Part model, mm, in its own coordinate system. A direction names the side the tool comes from. Give positions to 0.01 mm unless a question says otherwise; leave off trailing zeros. Loops run counter-clockwise (first coordinate to the right, second up) from the corner with the lowest first, then second, coordinate; pieces in that order, holes last. Notation, with made-up numbers: M 68,89.5 L 75,89.5 A22 ccw 75,125.5 Z; hole C 77.25,24 d7. An arc over 180 degrees is marked long. Put each result on its own line as item: value. Start each with the question number.
```python
from build123d import *

# Parameters (mm, degrees)
F1_DEPTH = 4


with BuildPart() as f1:
    # F0 (on Top) → F1 (new body)
    with BuildSketch(Plane.XY):
        with BuildLine():
            ThreePointArc((-21.3281772584, 26.4835794998), (-23.5728167331, 28.3513270209), (-20.7305210084, 27.6818181058))
            ThreePointArc((-20.7305210084, 27.6818181058), (-20.7359422147, 27.5544044904), (-20.7521666475, 27.4279118558))
            Line((-20.7521666475, 27.4279118558), (-19.7434481071, 27.4279118558))
            ThreePointArc((-19.7434481071, 27.4279118558), (-19.7337548746, 27.5547005483), (-19.7305210084, 27.6818181058))
            ThreePointArc((-19.7305210084, 27.6818181058), (-24.2927842524, 29.0949954876), (-21.3281772584, 25.3503430883))
            Line((-21.3281772584, 25.3503430883), (-21.3281772584, 26.4835794998))
        make_face()
        with BuildLine():
            ThreePointArc((-20.7521666475, 27.4279118558), (-20.949946226, 26.9007110538), (-21.3281772584, 26.4835794998))
            Line((-21.3281772584, 26.4835794998), (-21.3281772584, 25.3503430883))
            ThreePointArc((-21.3281772584, 25.3503430883), (-20.2427812606, 26.165608788), (-19.7434481071, 27.4279118558))
            Line((-19.7434481071, 27.4279118558), (-20.7521666475, 27.4279118558))
        make_face()
        with BuildLine():
            ThreePointArc((-19.7434481071, 27.4279118558), (-20.2427812606, 26.165608788), (-21.3281772584, 25.3503430883))
            Line((-21.3281772584, 25.3503430883), (-21.3281772584, -2.3181818942))
            Line((-21.3281772584, -2.3181818942), (-4.7461460084, -2.3181818942))
            Line((-4.7461460084, -2.3181818942), (-4.7461460084, 0.7742660224))
            Line((-4.7461460084, 0.7742660224), (-17.8711460084, 0.7742660224))
            Line((-17.8711460084, 0.7742660224), (-17.8711460084, 11.7182764391))
            Line((-17.8711460084, 11.7182764391), (-5.5404168417, 11.7182764391))
            Line((-5.5404168417, 11.7182764391), (-5.5404168417, 14.7716618558))
            Line((-5.5404168417, 14.7716618558), (-17.8711460084, 14.7716618558))
            Line((-17.8711460084, 14.7716618558), (-17.8711460084, 24.3549951891))
            Line((-17.8711460084, 24.3549951891), (-4.7461460084, 24.3549951891))
            Line((-4.7461460084, 24.3549951891), (-4.7461460084, 27.4279118558))
            Line((-4.7461460084, 27.4279118558), (-19.7434481071, 27.4279118558))
        make_face()
    extrude(amount=F1_DEPTH)


solid = f1.part
```
1) Band-saw the part on D-D on x = -23.25. Give the cut face in (y, z).
2) Band-saw the part on C-C on y = 6. Give the cut face in (x, z).
3) Pin check, flat tips, straight feed: pin 1 Ø1.2 at (x, z) = (-10.5, 1.5) entering from +Y; pin 2 Ø1.2 at (y, z) = (21, 1.5) entering from +X. Stop position of each tip, or through.
4) Band-saw the part on B-B on z = 3.55. Give the cut face in (x, y) (3 decimals), then the cut area to 3 significant figures.
5) Which spindle directions (+Z, -Z, +X, -X, +Y, -Y) get a long thin tool onto all of the face, cutting with end or side? Do faces 1 (the flat face through (-17.871, 19, 2)), 2 (the flat face through (-16, 14, 0)). Say none if no direction does.
6) Wall check: L1, parallel to Y at x = -11.75, z = 2.8 (3 decimals); L2, parallel to X at y = 24, z = 2.1; L3, parallel to Y at x = -23, z = 2.2. Give the ranges that are in metal, low to high.
7) Band-saw the part on A-A on x = -15. Give the cut face in (y, z) (3 decimals).
8) Mould opens along Y. For faces 3 (the flat face through (-13, -2.318, 2)), 4 (the flat face through (-5.54, 13, 2)), 5 (the flat face through (-4.746, 26, 2)) say: +Y half, -Y half, draft (parallel to the pull), parting line (faces both ways), or undercut.
Evaluation:
1. outline: M 25.4,0 L 26.58,0 L 26.58,4 L 25.4,4 Z; M 28.78,0 L 29.96,0 L 29.96,4 L 28.78,4 Z
2. outline: M -21.33,0 L -17.87,0 L -17.87,4 L -21.33,4 Z
3. pin 1: y = 27.43
3. pin 2: x = -17.87
4. outline: M -21.328,-2.318 L -4.746,-2.318 L -4.746,0.774 L -17.871,0.774 L -17.871,11.718 L -5.54,11.718 L -5.54,14.772 L -17.871,14.772 L -17.871,24.355 L -4.746,24.355 L -4.746,27.428 L -19.743,27.428 A2.5 ccw long -21.328,25.35 Z; hole C -22.231,27.682 d3
4. area: 232 mm2
5. face 1: +Z, -Z, +X
5. face 2: -Z, +X, -X, +Y, -Y
6. L1: -2.318 to 0.774, 11.718 to 14.772, 24.355 to 27.428
6. L2: -21.33 to -17.87
6. L3: 25.3 to 26.39, 28.97 to 30.06
7. outline: M -2.318,0 L 0.774,0 L 0.774,4 L -2.318,4 Z; M 11.718,0 L 14.772,0 L 14.772,4 L 11.718,4 Z; M 24.355,0 L 27.428,0 L 27.428,4 L 24.355,4 Z
8. face 3: -Y half
8. face 4: undercut
8. face 5: draft
